Design review of the part built by this model. Coordinates are the model's own, in mm. A direction names the side the tool comes from. Coordinates: 2 decimals unless noted, no trailing zeros. Loops run counter-clockwise (first coordinate to the right, second up) from the corner with the lowest first, then second, coordinate; pieces in that order, holes last. Notation, with made-up numbers: M 7.25,54.5 L 48.25,54.5 A17 ccw 48.25,59.5 Z; hole C 84,-12.5 d10. An arc over 180 degrees is marked long. Put each result on its own line as item: value. Start each with the question number.
(1) Take a section at B-B, the plane y = -2.25. Give the boundary of the cut face in (x, z).
(2) For faces 1 (the cylindrical face through (-1.08, 4.88, 112.51)), 2 (the cylindrical face through (-0.59, 4.46, 224.3)), 3 (the cylindrical face through (0.59, 4.46, 3.7)), list the 3-axis set-ups (+Z, -Z, +X, -X, +Y, -Y) from which the entire face can be reached by the end or side of a thin tool; tool diameter is ignored.
(3) Take a section at A-A, the plane x = 1.25. Give the boundary of the cut face in (y, z).
(4) For probe 1 along X at (y, z) = (-0.25, 213); probe 2 along Z at (x, y) = (-3.5, -3); probe 3 along Y at (x, z) = (-0.5, 62), list the stretches that pass through material, from the lowest coordinate up. Write a range as [from, to].
(5) Clearance check with flat-ended pins moving along their axes: pin 1 (1.5 mm diameter, centred on y = -2, z = 79.5, fed in from -X); pin 2 (5 mm diameter, centred on x = -3, z = 97, fed in from +Y). State where each tip first meets the part, or that it passes through.
(6) Take a section at C-C, the plane z = 173. Give the boundary of the cut face in (x, y).
Autodesk Inventor part; units mm, degrees
ref_plane "YZ Plane" through (0, 0, 0) normal (1, 0, 0) x (0, 1, 0)
ref_plane "XZ Plane" through (0, 0, 0) normal (0, 1, 0) x (-1, 0, 0)
ref_plane "XY Plane" through (0, 0, 0) normal (0, 0, 1) x (1, 0, 0)
sketch "Sketch2" plane through (0, 0, 0) normal (0, 0, 1) x (1, 0, 0)
  circle A0 centre (0, 0) radius 5
  dimension "d7" = 10
extrude "Extrusion2" add sketch "Sketch2" along normal blind 228
sketch "Sketch3" plane through (0, 0, 228) normal (0, 0, 1) x (1, 0, 0)
  circle A0 centre (0, 0) radius 4.5
  circle A1 centre (0, 0) radius 5
  dimension "d10" = 9
extrude "Extrusion3" cut sketch "Sketch3" against normal blind 7.5
sketch "Sketch4" plane through (0, 0, 0) normal (0, 0, -1) x (-1, 0, 0)
  circle A0 centre (0, 0) radius 4.5
  circle A1 centre (0, 0) radius 5
  dimension "d13" = 9
  dimension "d14" = 10
extrude "Extrusion4" cut sketch "Sketch4" against normal blind 7.5
equation "\"BendRadius\" = Thickness"
equation "\"BendReliefWidth\" = Thickness"
equation "\"BendReliefDepth\" = 0.5 * Thickness"
equation "\"CornerReliefSize\" = 4 * Thickness"
equation "\"MinimumRemnant\" = 2 * Thickness"
equation "\"TransitionRadius\" = BendRadius"
equation "\"JacobiRadiusSize\" = BendRadius"
equation "\"GapSize\" = Thickness"
properties part number "link2"
Computed values:
1. outline: M -4.47,7.5 L -3.9,7.5 L -3.9,0 L 3.9,0 L 3.9,7.5 L 4.47,7.5 L 4.47,220.5 L 3.9,220.5 L 3.9,228 L -3.9,228 L -3.9,220.5 L -4.47,220.5 Z
2. face 1: +Z, -Z
2. face 2: +Z
2. face 3: -Z
3. outline: M -4.84,7.5 L -4.32,7.5 L -4.32,0 L 4.32,0 L 4.32,7.5 L 4.84,7.5 L 4.84,220.5 L 4.32,220.5 L 4.32,228 L -4.32,228 L -4.32,220.5 L -4.84,220.5 Z
4. probe 1: x = [-4.99, 4.99]
4. probe 2: z = [7.5, 220.5]
4. probe 3: y = [-4.97, 4.97]
5. pin 1: stops at x = -4.84
5. pin 2: stops at y = 4.97
6. outline: C 0,0 d10
